from build123d import *

# Parameters (mm, degrees)
SKETCH_1_W             = 420
SKETCH_1_H             = 304.2
SKETCH_1_R             = 2.55
EXTRUDE_1_DEPTH        = 4
SKETCH_2_R             = 1.6
SKETCH_2_W             = 45
SKETCH_2_H             = 80
CUT_EXTRUDE_1_DEPTH    = 260.326840107
SKETCH_4_R             = 2.15
CUT_EXTRUDE_3_DEPTH    = 260.326840107
PATTERN_LINEAR_3_COUNT = 4
PATTERN_LINEAR_3_PITCH = 95
SKETCH_7_R             = 2.15
SKETCH_7_R_2           = 1.6
CUT_EXTRUDE_5_DEPTH    = 260.326840107
SKETCH_9_R             = 2.15
EXTRUDE_2_DEPTH        = 4
FILLET_1_R             = 10


with BuildPart() as part:
    # 草图1 → 凸台-拉伸1 (new body)
    with BuildSketch(Plane(origin=(0, 0, 0), x_dir=(1, 0, 0), z_dir=(0, 1, 0))):
        Rectangle(SKETCH_1_W, SKETCH_1_H)
        with Locations(Location((-19, -144.1, 0), (0, 0, 270))):
            Circle(SKETCH_1_R, mode=Mode.SUBTRACT)
        with Locations(Location((19, -144.1, 0), (0, 0, 270))):
            Circle(SKETCH_1_R, mode=Mode.SUBTRACT)
    extrude(amount=EXTRUDE_1_DEPTH)

    # 草图2 → 切除-拉伸1 (cut, through all)
    with BuildSketch(Plane(origin=(0, 0, 0), x_dir=(1, 0, 0), z_dir=(0, 1, 0))):
        with Locations(Location((-147, 92.1, 0), (0, 0, 270))):
            Circle(SKETCH_2_R)
        with Locations(Location((-147, 62.1, 0), (0, 0, 270))):
            Circle(SKETCH_2_R)
        with Locations(Location((-123.6, 62.1, 0), (0, 0, 270))):
            Circle(SKETCH_2_R)
        with Locations(Location((-123.6, 92.1, 0), (0, 0, 270))):
            Circle(SKETCH_2_R)
        with Locations((-187.5, 77.1)):
            Rectangle(SKETCH_2_W, SKETCH_2_H)
    cut_extrude_1 = extrude(amount=CUT_EXTRUDE_1_DEPTH, mode=Mode.SUBTRACT)

    # 镜向1: 切除-拉伸1 across plane
    add(cut_extrude_1.mirror(Plane(origin=(0, 0, 0), x_dir=(0, 0, 1), z_dir=(1, 0, 0))), mode=Mode.SUBTRACT)

    # 草图4 → 切除-拉伸3 (cut, through all)
    with BuildSketch(Plane(origin=(0, 0, 0), x_dir=(1, 0, 0), z_dir=(0, 1, 0))):
        with Locations(Location((-125, 142.1, 0), (0, 0, 270))):
            Circle(SKETCH_4_R)
        with Locations(Location((125, 142.1, 0), (0, 0, 270))):
            Circle(SKETCH_4_R)
        with Locations(Location((0, 142.1, 0), (0, 0, 270))):
            Circle(SKETCH_4_R)
    cut_extrude_3 = extrude(amount=CUT_EXTRUDE_3_DEPTH, mode=Mode.SUBTRACT)

    # 阵列(线性)3: 切除-拉伸3 ×4
    with Locations(*[(0, 0, i * PATTERN_LINEAR_3_PITCH) for i in range(1, PATTERN_LINEAR_3_COUNT)]):
        add(cut_extrude_3, mode=Mode.SUBTRACT)

    # 草图7 → 切除-拉伸5 (cut, through all)
    with BuildSketch(Plane(origin=(0, 0, 0), x_dir=(1, 0, 0), z_dir=(0, 1, 0))):
        with Locations(Location((-200, 22.1, 0), (0, 0, 270))):
            Circle(SKETCH_7_R)
        with Locations(Location((-200, -137.9, 0), (0, 0, 270))):
            Circle(SKETCH_7_R)
        with Locations(Location((-200, -57.9, 0), (0, 0, 270))):
            Circle(SKETCH_7_R)
        with Locations(Location((200, -57.9, 0), (0, 0, 270))):
            Circle(SKETCH_7_R)
        with Locations(Location((200, 22.1, 0), (0, 0, 270))):
            Circle(SKETCH_7_R)
        with Locations(Location((200, -137.9, 0), (0, 0, 270))):
            Circle(SKETCH_7_R)
        with Locations(Location((-171.25, 142.1, 0), (0, 0, 270))):
            Circle(SKETCH_7_R_2)
        with Locations(Location((171.25, 142.1, 0), (0, 0, 270))):
            Circle(SKETCH_7_R_2)
        with Locations((171.25, -257.9)):
            Circle(SKETCH_7_R_2)
        with Locations((-171.25, -257.9)):
            Circle(SKETCH_7_R_2)
    extrude(amount=CUT_EXTRUDE_5_DEPTH, mode=Mode.SUBTRACT)

    # 草图9 → 凸台-拉伸2 (add, through all)
    with BuildSketch(Plane(origin=(0, 0, 0), x_dir=(1, 0, 0), z_dir=(0, 1, 0))):
        with Locations((0, -142.9)):
            Circle(SKETCH_9_R)
    extrude(amount=EXTRUDE_2_DEPTH)

    # 圆角1
    fillet_1_edges = [part.edges().sort_by_distance(p)[0] for p in [
        (-210, 2, -117.1),
        (-210, 2, -37.1),
        (210, 2, -37.1),
        (210, 2, -117.1),
        (-210, 2, -152.1),
        (210, 2, -152.1),
        (210, 2, 152.1),
        (-210, 2, 152.1),
    ]]
    fillet(fillet_1_edges, radius=FILLET_1_R)


solid = part.part
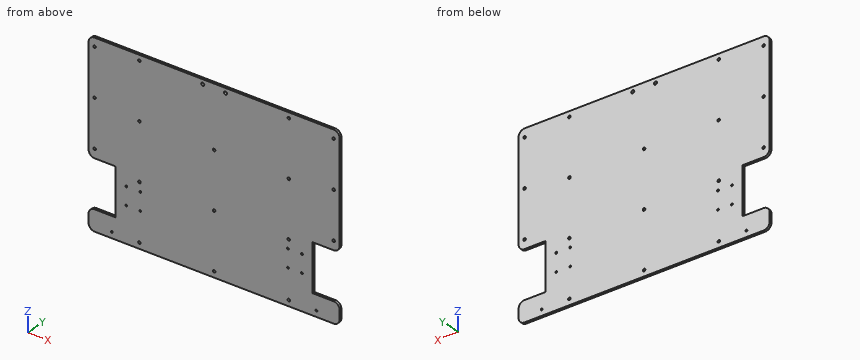
Part model, mm, in its own coordinate system. Coordinates: 2 decimals unless noted, no trailing zeros.
(1) Slice it at A-A, the plane y = 0.8. State how many separate pieces and enclosed holes the cut face has, and give its area (3 significant figures).
Check sheet entries:
separate pieces: 1
enclosed holes: 29
area: 120,000 mm2
(2) Probe L1, parallel to Z at x = 0, y = 1.7; L2, parallel to Z at x = 171.25, y = 3.1; L3, parallel to X at y = 2.75, z = 57.9. List the from-to ranges inside material, lowest first.
Check sheet entries:
L1: z = -152.1 to -144.25, -139.95 to -49.25, -44.95 to 45.75, 50.05 to 152.1
L2: z = -152.1 to -143.7, -140.5 to -117.1, -37.1 to 152.1
L3: x = -210 to -202.15, -197.85 to 197.85, 202.15 to 210
(3) Pin check, flat tips, straight feed: pin 1 Ø1.9 at (x, z) = (147, -92.1) entering from -Y; pin 2 Ø2 at (y, z) = (3.5, -64) entering from +X. Stop position of each tip, or through.
Check sheet entries:
pin 1: passes through
pin 2: stops at x = 165
